The model under review builds one solid part; all positions refer to its coordinate system, in mm. A direction names the side the tool comes from. Give positions to 0.01 mm unless a question says otherwise; leave off trailing zeros. Order: outer loops, then holes, each group sorted by start corner. A loop starts at its lowest first (then second) coordinate and runs counter-clockwise, first axis right, second up. Notation, with made-up numbers: (-12.75, 86) - (13.25, 86) arc R22 cw to (13.25, 92) - close; hole circle Ø1 at (7.25, 86). An arc over 180 degrees is marked (long way). Use CSV: the item, a comma, the result in double quotes.
```python
from build123d import *

# Parameters (mm, degrees)
SKETCH1_R           = 2.5
BOSS_EXTRUDE1_DEPTH = 5
SKETCH2_W           = 3
SKETCH2_H           = 70
CUT_EXTRUDE3_DEPTH  = 10
SKETCH7_W           = 3
SKETCH7_H           = 5
BOSS_EXTRUDE5_DEPTH = 7
SKETCH8_R           = 0.5
CUT_EXTRUDE5_DEPTH  = 40
SKETCH9_W           = 120
SKETCH9_H           = 3
BOSS_EXTRUDE6_DEPTH = 30
SKETCH10_R          = 2.5
CUT_EXTRUDE6_DEPTH  = 100


with BuildPart() as part:
    # Sketch1 → Boss-Extrude1 (new body)
    with BuildSketch(Plane.XY):
        Polygon((-50, 20), (-60, 20), (-60, 0), (-50, 0), (-50, -5), (-60, -5), (-60, -25), (-50, -25), (-50, -30), (-60, -30), (-60, -50), (-50, -50), (-50, -55), (-57, -55), (-57, -65), (-32, -65), (-32, -75), (33, -60), (33, -55), (-10, -55), (-10, -50), (0, -50), (0, -30), (-10, -30), (-10, -25), (0, -25), (0, -5), (-10, -5), (-10, 0), (0, 0), (0, 20), (-10, 20), (-10, 28), (-50, 28), align=None)
        with Locations((-42.5, 22.5)):
            Circle(SKETCH1_R, mode=Mode.SUBTRACT)
        with Locations((-17.5, 22.5)):
            Circle(SKETCH1_R, mode=Mode.SUBTRACT)
        with Locations((-42.5, -2.5)):
            Circle(SKETCH1_R, mode=Mode.SUBTRACT)
        with Locations((-17.5, -2.5)):
            Circle(SKETCH1_R, mode=Mode.SUBTRACT)
        with Locations((-17.5, -27.5)):
            Circle(SKETCH1_R, mode=Mode.SUBTRACT)
        with Locations((-42.5, -27.5)):
            Circle(SKETCH1_R, mode=Mode.SUBTRACT)
        with Locations((-17.5, -52.5)):
            Circle(SKETCH1_R, mode=Mode.SUBTRACT)
        with Locations((-42.5, -52.5)):
            Circle(SKETCH1_R, mode=Mode.SUBTRACT)
    extrude(amount=BOSS_EXTRUDE1_DEPTH)

    # Sketch2 → Cut-Extrude3 (cut)
    with BuildSketch(Plane(origin=(0, 0, 0), x_dir=(-1, 0, 0), z_dir=(0, 0, -1))):
        with Locations((58.5, -15)):
            Rectangle(SKETCH2_W, SKETCH2_H)
        with Locations((1.5, -15)):
            Rectangle(SKETCH2_W, SKETCH2_H)
    extrude(amount=-CUT_EXTRUDE3_DEPTH, mode=Mode.SUBTRACT)

    # Sketch7 → Boss-Extrude5 (add)
    with BuildSketch(Plane(origin=(14.814606742, -64.196629213, 0), x_dir=(0.97439119569462, 0.22485950669875845, 0), z_dir=(0.22485950669875845, -0.97439119569462, 0))):
        with Locations((-46.544981265, 2.5)):
            Rectangle(SKETCH7_W, SKETCH7_H)
        with Locations((-13.544981265, 2.5)):
            Rectangle(SKETCH7_W, SKETCH7_H)
    extrude(amount=BOSS_EXTRUDE5_DEPTH)

    # Sketch8 → Cut-Extrude5 (cut)
    with BuildSketch(Plane(origin=(-46.814606742, -10.803370787, 0), x_dir=(0, 0, 1), z_dir=(-0.97439119569462, -0.22485950669875848, 0))):
        with Locations(Location((2.5, -70.383835463, 0), (0, 0, 270))):
            Circle(SKETCH8_R)
    extrude(amount=-CUT_EXTRUDE5_DEPTH, mode=Mode.SUBTRACT)

    # Sketch9 → Boss-Extrude6 (add)
    with BuildSketch(Plane.XY.offset(5)):
        with Locations((3, -56.5)):
            Rectangle(SKETCH9_W, SKETCH9_H)
        with Locations((3, 18.5)):
            Rectangle(SKETCH9_W, SKETCH9_H)
    extrude(amount=BOSS_EXTRUDE6_DEPTH)

    # Sketch10 → Cut-Extrude6 (cut)
    with BuildSketch(Plane.XZ.offset(58)):
        with Locations((48, 20)):
            Circle(SKETCH10_R)
        Polygon((-57, 20), (3, 35), (-57, 35), align=None)
    extrude(amount=-CUT_EXTRUDE6_DEPTH, mode=Mode.SUBTRACT)


solid = part.part
```
Item 1: Take a section at D-D, the plane z = 31. Give the boundary of the cut face in (x, y), and give its area (3 significant figures).
Results list:
outline,"(-13, -58) - (63, -58) - (63, -55) - (-13, -55) - close; (-13, 17) - (63, 17) - (63, 20) - (-13, 20) - close"
area,"456 mm2"
Item 2: Tool access review of faces 1 (the face through (-53, -5, 2)), 2 (the face through (-45, -65, 2)), 3 (the face through (-6, -30, 2)), 4 (the face through (48, -56, 5)): name each direction out of +Z, -Z, +X, -X, +Y, -Y from which nothing blocks a thin tool from reaching the whole face with its end or side.
Results list:
face 1,"+Z, -Z, -X"
face 2,"+Z, -Z, -X, -Y"
face 3,"+Z, -Z, +X"
face 4,"-Z, +X, +Y, -Y"
Item 3: Take a section at B-B, the plane z = 16. Give the boundary of the cut face in (x, y).
Results list:
outline,"(-57, -58) - (63, -58) - (63, -55) - (-57, -55) - close; (-57, 17) - (63, 17) - (63, 20) - (-57, 20) - close"
Item 4: Clearance check with flat-ended pins moving along their axes: pin 1 (2.5 mm diameter, centred on y = -27, z = 3.5, fed in from -X); pin 2 (4 mm diameter, centred on x = -53.5, z = 3.5, fed in from -Y); pin 3 (4 mm diameter, centred on x = 48, z = 20, fed in from +Y); pin 4 (0.9 mm diameter, centred on x = 46.5, y = 19, fed in from -Z). State where each tip first meets the part, or that it passes through.
Results list:
pin 1,"stops at x = -50"
pin 2,"stops at y = -65"
pin 3,"passes through"
pin 4,"stops at z = 5"
Item 5: Mouldability with a two-part tool opening along Y and no side actions: class faces 5 (the face through (-30, 24, 5)), 6 (the face through (2, -55, 17)), 7 (the face through (3.17, -74.068, 2.535)), 8 (the face through (-19.5, -54, 2.5)) as pulls with the +Y half, pulls with the -Y half, needs draft (parallel to the pull), parting line crosses it, or undercut.
Results list:
face 5,"needs draft"
face 6,"undercut"
face 7,"pulls with the -Y half"
face 8,"undercut"
Item 6: Wall thickness on L1, parallel to Y at x = -42.5, z = 2.4; L2, parallel to Z at x = 48, y = -56.1; L3, parallel to Y at x = -42, z = 2: over which ranges is each line inside the solid? List them lowest first.
Results list:
L1,"y = -65 to -55, -50 to -30, -25 to -5, 0 to 20, 25 to 28"
L2,"z = 5 to 17.5, 22.5 to 35"
L3,"y = -65 to -54.95, -50.05 to -29.95, -25.05 to -4.95, -0.05 to 20.05, 24.95 to 28"
Item 7: Take a section at A-A, the plane x = 48. Give the boundary of the cut face in (y, z).
Results list:
outline,"(-58, 5) - (-55, 5) - (-55, 17.5) - (-58, 17.5) - close; (-58, 22.5) - (-55, 22.5) - (-55, 35) - (-58, 35) - close; (17, 5) - (20, 5) - (20, 17.5) - (17, 17.5) - close; (17, 22.5) - (20, 22.5) - (20, 35) - (17, 35) - close"
Item 8: Take a section at C-C, the plane y = -27.5. Give the boundary of the cut face in (x, z).
Results list:
outline,"(-50, 0) - (-45, 0) - (-45, 5) - (-50, 5) - close; (-40, 0) - (-20, 0) - (-20, 5) - (-40, 5) - close; (-15, 0) - (-10, 0) - (-10, 5) - (-15, 5) - close"
